Study the drawing (mm; zero at the part's minimum x, y, z) and answer. A direction names the side the tool comes from. Round coordinates to 2 decimals unless told otherwise and drop trailing zeros. Order: outer loops, then holes, each group sorted by start corner. A loop starts at its lowest first (then second) coordinate and runs counter-clockwise, first axis right, second up. Notation, with made-up numbers: (36, 22) - (87, 22) arc R17 ccw to (87, 55) - close; hole circle Ø1 at (30, 89). An arc over 180 degrees is marked (long way). Put each result on its own line as item: value.
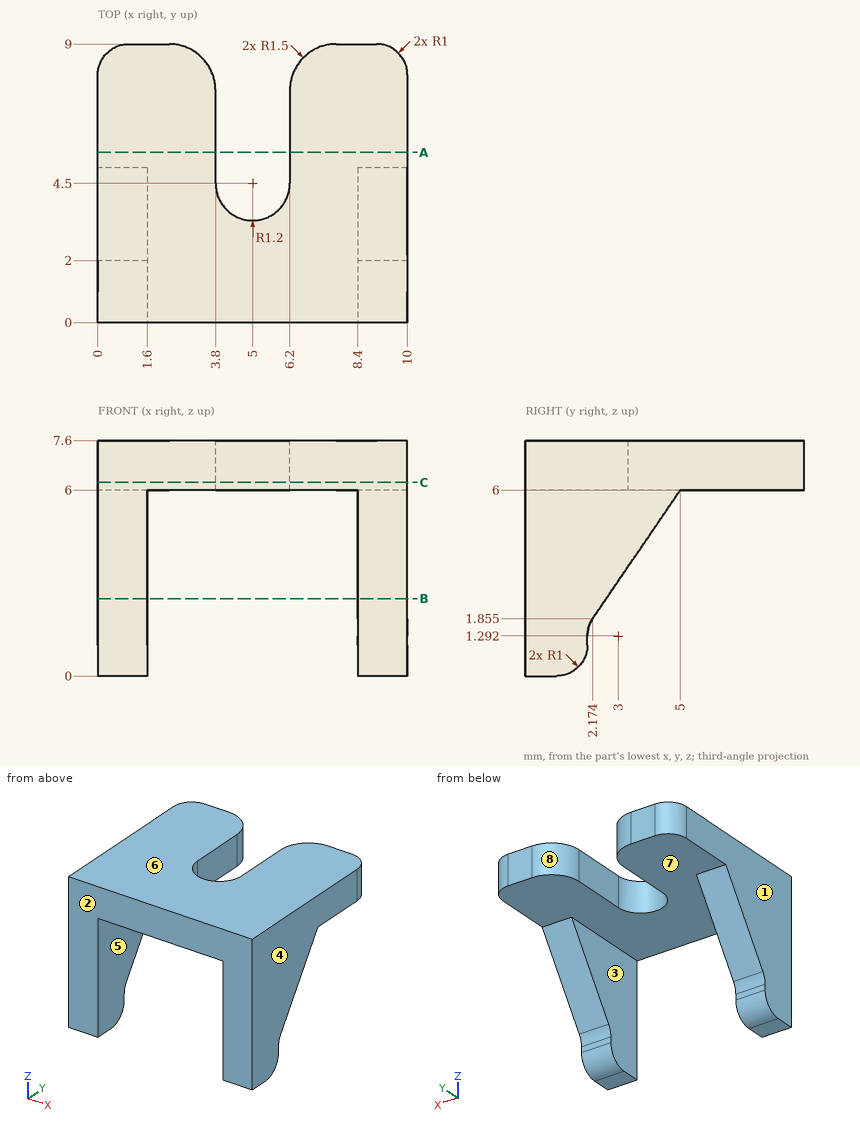
1) For the marked faces 5, 6, 7 and 8, determine the directions among +Z, -Z, +X, -X, +Y, -Y from which every point of the face is accessible in a straight line to the end or side of a thin tool.
Findings below:
face 5: -Z, +Y, -Y
face 6: +Z, +X, -X, +Y, -Y
face 7: -Z, +Y
face 8: +Z, -Z, +Y
2) A cutting plane is placed at A-A on y = 5.5. Write down the section's boundary in (x, z).
Findings below:
outline: (0, 6) - (3.8, 6) - (3.8, 7.6) - (0, 7.6) - close; (6.2, 6) - (10, 6) - (10, 7.6) - (6.2, 7.6) - close
3) Straight lines are drawn through the part: L1, parallel to X at y = 2.5, z = 5.25; L2, parallel to Z at x = 7.75, y = 6.5; L3, parallel to Y at x = 3.5, z = 6.5. For each, find the intervals that lie inside material, in ascending order. Write a range as from..to.
Findings below:
L1: x = 0..1.6, 8.4..10
L2: z = 6..7.6
L3: y = 0..8.4
4) A cutting plane is placed at B-B on z = 2.5. Write down the section's boundary in (x, y).
Findings below:
outline: (0, 0) - (1.6, 0) - (1.6, 2.61) - (0, 2.61) - close; (8.4, 0) - (10, 0) - (10, 2.61) - (8.4, 2.61) - close
5) A cutting plane is placed at C-C on z = 6.25. Write down the section's boundary in (x, y).
Findings below:
outline: (0, 0) - (10, 0) - (10, 8) arc R1 ccw to (9, 9) - (7.7, 9) arc R1.5 ccw to (6.2, 7.5) - (6.2, 4.5) arc R1.2 cw to (3.8, 4.5) - (3.8, 7.5) arc R1.5 ccw to (2.3, 9) - (1, 9) arc R1 ccw to (0, 8) - close
6) Given pin 1 Ø1 at (x, z) = (5.5, 4) entering from +Y; pin 2 Ø3 at (x, y) = (6.5, 2) entering from -Z; pin 3 Ø4 at (x, z) = (3, 2.5) entering from +Y, each flat-ended and moving along its own axis, determine where each tip first touches the part or whether it passes through.
Findings below:
pin 1: passes through
pin 2: stops at z = 6
pin 3: stops at y = 3.59
7) For a pull along X with two mould halves and no side action, classify the marked faces 1, 2, 3 and 4 as pulls with the +X half, pulls with the -X half, needs draft (parallel to the pull), parting line crosses it, or undercut.
Findings below:
face 1: pulls with the -X half
face 2: needs draft
face 3: undercut
face 4: pulls with the +X half
